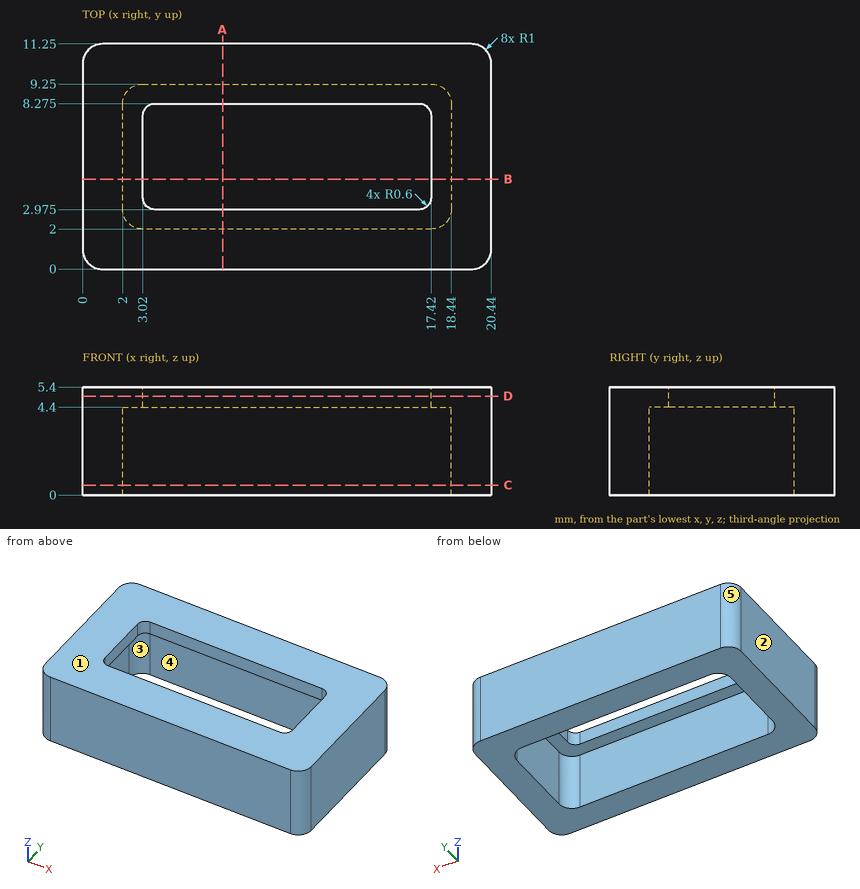
Input: dimensioned drawing with shaded views. Units: mm. Origin: part minimum x, y, z. A direction names the side the tool comes from. Give positions to 0.01 mm unless a question says otherwise; leave off trailing zeros. Loops run counter-clockwise (first coordinate to the right, second up) from the corner with the lowest first, then second, coordinate; pieces in that order, holes last. Notation, with made-up numbers: (25, -7) - (82, -7) arc R25 ccw to (82, 28) - close; hole circle Ø9 at (28.25, -39.5). An arc over 180 degrees is marked (long way). Answer as CSV lines item,"result". Start each with the question number.
(1) Section query C-C (z = 0.5). Output: boundary loops of the cut face in (x, y), and give its area (3 significant figures).
(2) Pin query (flat end, axial travel): P1, Ø1.1, axis at y = 5, z = 5, coming from the -X side; P2, Ø3.5, axis at x = 7.5, y = 5.5, coming from the -Z side. Return the tip coordinate at first contact, or that it passes through.
(3) Mould query, pull axis X, two halves, no side actions, for the marked faces 1, 2 and 3. Classes: +X half, -X half, draft (parallel to the pull), parting line (faces both ways), or undercut.
(4) Section query D-D (z = 4.95). Output: boundary loops of the cut face in (x, y) (3 decimals).
(5) Section query B-B (y = 4.5). Output: boundary loops of the cut face in (x, z).
(6) Section query A-A (x = 7). Output: boundary loops of the cut face in (y, z) (3 decimals), and give its area (4 significant figures).
(7) Ray query, line 1 along Y through (x, z) = (13, 5.2) (3 decimals); line 2 along X through (y, z) = (4.25, 0.75); line 3 along Y through (x, z) = (3.75, 1.3). Return the intervals inside material, ascending. Write a range as [from, to].
(8) Reachability of the marked faces 4 and 5 from +Z, -Z, +X, -X, +Y, -Y: full face, straight path, thin tool, end or side. Return the list, or none.
Worked answers:
1,outline,"(0, 1) arc R1 ccw to (1, 0) - (19.44, 0) arc R1 ccw to (20.44, 1) - (20.44, 10.25) arc R1 ccw to (19.44, 11.25) - (1, 11.25) arc R1 ccw to (0, 10.25) - close; hole (2, 3) arc R1 ccw to (3, 2) - (17.44, 2) arc R1 ccw to (18.44, 3) - (18.44, 8.25) arc R1 ccw to (17.44, 9.25) - (3, 9.25) arc R1 ccw to (2, 8.25) - close"
1,area,"111 mm^2"
2,P1,"stops at x = 0"
2,P2,"passes through"
3,face 1,"draft"
3,face 2,"-X half"
3,face 3,"undercut"
4,outline,"(0, 1) arc R1 ccw to (1, 0) - (19.44, 0) arc R1 ccw to (20.44, 1) - (20.44, 10.25) arc R1 ccw to (19.44, 11.25) - (1, 11.25) arc R1 ccw to (0, 10.25) - close; hole (3.02, 3.575) arc R0.6 ccw to (3.62, 2.975) - (16.82, 2.975) arc R0.6 ccw to (17.42, 3.575) - (17.42, 7.675) arc R0.6 ccw to (16.82, 8.275) - (3.62, 8.275) arc R0.6 ccw to (3.02, 7.675) - close"
5,outline,"(0, 0) - (2, 0) - (2, 4.4) - (3.02, 4.4) - (3.02, 5.4) - (0, 5.4) - close; (17.42, 4.4) - (18.44, 4.4) - (18.44, 0) - (20.44, 0) - (20.44, 5.4) - (17.42, 5.4) - close"
6,outline,"(0, 0) - (2, 0) - (2, 4.4) - (2.975, 4.4) - (2.975, 5.4) - (0, 5.4) - close; (8.275, 4.4) - (9.25, 4.4) - (9.25, 0) - (11.25, 0) - (11.25, 5.4) - (8.275, 5.4) - close"
6,area,"23.55 mm^2"
7,line 1,"y = [0, 2.975], [8.275, 11.25]"
7,line 2,"x = [0, 2], [18.44, 20.44]"
7,line 3,"y = [0, 2], [9.25, 11.25]"
8,face 4,"-Z"
8,face 5,"+Z, -Z, -X, +Y"
